Part print with two shaded views. Sizes in mm from the minimum x, y, z corner. Coordinates: 2 decimals unless noted, no trailing zeros. Write each loop counter-clockwise with the first axis right and the second up, starting at its lowest first coordinate (ties: lowest second). Pieces come first, ordered by that corner, then holes.
Q1. Drill centre lines: probe 1 along Y at (x, z) = (63.5, 1.35); probe 2 along X at (y, z) = (10, 2.55); probe 3 along X at (y, z) = (12, 1.15). Where is each one in solid material? Low to high.
Q2. Pin check, flat tip, straight feed: P1, Ø8, axis at x = 45, y = 12.5, coming from the +Z side. Stop position of the tip, or through.
Q3. Band-saw the part on A-A, the plane y = 12.5. Write the cut outline in (x, z), plus the area to 3 significant figures.
Q4. Band-saw the part on C-C, the plane y = 8.5. Write the cut outline in (x, z).
Q5. Band-saw the part on B-B, the plane x = 63.5. Write the cut outline in (y, z), plus the area to 3 significant figures.
Q6. Band-saw the part on D-D, the plane z = 2.15. Write the cut outline in (x, y), plus the area to 3 significant figures.
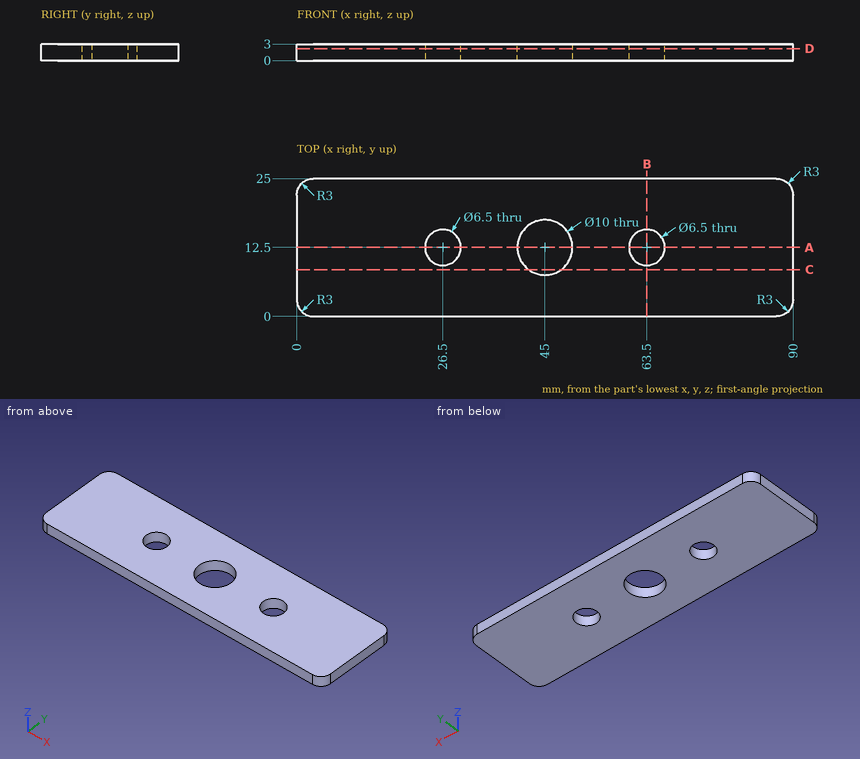
Answer sheet:
1. probe 1: y = 0 to 9.25, 15.75 to 25
1. probe 2: x = 0 to 24.42, 28.58 to 40.67, 49.33 to 61.42, 65.58 to 90
1. probe 3: x = 0 to 23.29, 29.71 to 40.03, 49.97 to 60.29, 66.71 to 90
2. P1: passes through
3. outline: (0, 0) - (23.25, 0) - (23.25, 3) - (0, 3) - close; (29.75, 0) - (40, 0) - (40, 3) - (29.75, 3) - close; (50, 0) - (60.25, 0) - (60.25, 3) - (50, 3) - close; (66.75, 0) - (90, 0) - (90, 3) - (66.75, 3) - close
3. area: 201 mm2
4. outline: (0, 0) - (42, 0) - (42, 3) - (0, 3) - close; (48, 0) - (90, 0) - (90, 3) - (48, 3) - close
5. outline: (0, 0) - (9.25, 0) - (9.25, 3) - (0, 3) - close; (15.75, 0) - (25, 0) - (25, 3) - (15.75, 3) - close
5. area: 55.5 mm2
6. outline: (0, 3) arc R3 ccw to (3, 0) - (87, 0) arc R3 ccw to (90, 3) - (90, 22) arc R3 ccw to (87, 25) - (3, 25) arc R3 ccw to (0, 22) - close; hole circle Ø6.5 at (26.5, 12.5); hole circle Ø10 at (45, 12.5); hole circle Ø6.5 at (63.5, 12.5)
6. area: 2,100 mm2
